Input: part model. Units: mm. Frame: model coordinates. A direction names the side the tool comes from. Round coordinates to 2 decimals unless told otherwise and drop trailing zeros. Loops run counter-clockwise (first coordinate to the right, second up) from the corner with the lowest first, then second, coordinate; pieces in that order, holes last. Notation, with made-up numbers: (83, 26.5) - (91, 26.5) arc R15 cw to (91, 34.5) - close; hole circle Ø9 at (86.25, 26). An arc over 180 degrees is marked (long way). One line per question, with ' | ' between items. Start each with the question number.
from build123d import *

# Parameters (mm, degrees)
F0_W     = 76.2
F0_H     = 76.2
F0_W_2   = 73.025
F0_H_2   = 73.025
F1_DEPTH = 668.3375
F2_R     = 5.08
F3_R     = 5.08
F4_R     = 5.08
F5_R     = 5.08
F6_R     = 5.08
F7_R     = 5.08


with BuildPart() as f1:
    # F0 (on Top) → F1 (new body)
    with BuildSketch(Plane.XY):
        Rectangle(F0_W, F0_H)
        Rectangle(F0_W_2, F0_H_2, mode=Mode.SUBTRACT)
    extrude(amount=F1_DEPTH)

    # F2
    f2_edges = [f1.edges().sort_by_distance(p)[0] for p in [
        (-38.1, -38.1, 334.16875),
    ]]
    fillet(f2_edges, radius=F2_R)

    # F3
    f3_edges = [f1.edges().sort_by_distance(p)[0] for p in [
        (38.1, -38.1, 334.16875),
        (38.1, 38.1, 334.16875),
    ]]
    fillet(f3_edges, radius=F3_R)

    # F4
    f4_edges = [f1.edges().sort_by_distance(p)[0] for p in [
        (-36.5125, 36.5125, 334.16875),
    ]]
    fillet(f4_edges, radius=F4_R)

    # F5
    f5_edges = [f1.edges().sort_by_distance(p)[0] for p in [
        (-38.1, 38.1, 334.16875),
        (36.5125, -36.5125, 334.16875),
    ]]
    fillet(f5_edges, radius=F5_R)

    # F6
    f6_edges = [f1.edges().sort_by_distance(p)[0] for p in [
        (-36.5125, -36.5125, 334.16875),
    ]]
    fillet(f6_edges, radius=F6_R)

    # F7
    f7_edges = [f1.edges().sort_by_distance(p)[0] for p in [
        (36.5125, 36.5125, 334.16875),
    ]]
    fillet(f7_edges, radius=F7_R)


solid = f1.part
(1) Reachability of faces 4 (the face through (38.1, 0, 329)), 5 (the face through (36.512, 0, 329)) from +Z, -Z, +X, -X, +Y, -Y: full face, straight path, thin tool, end or side. Return the list, or none.
(2) Pull-direction query (Y, two-part tool) for faces 1 (the face through (-38.1, 0, 329)), 2 (the face through (-36.512, 0, 329)), 3 (the face through (0, 38.1, 329)); classes: released by +Y, released by -Y, zero draft, split by the parting line, or undercut.
(3) Section A-A, the plane y = 0.5. Output: boundary loops of the cut face in (x, z).
(4) Line query: line 1 along Y through (x, z) = (-24.5, 444); line 2 along X through (y, z) = (35, 199). Output: solid intervals per line, ascending. Write a range as from..to.
(5) Section C-C, the plane z = 69. Output: boundary loops of the cut face in (x, y).
Derived:
1) face 4: +Z, -Z, +X, +Y, -Y | face 5: +Z, -Z
2) face 1: zero draft | face 2: undercut | face 3: released by +Y
3) outline: (-38.1, 0) - (-36.51, 0) - (-36.51, 668.34) - (-38.1, 668.34) - close; (36.51, 0) - (38.1, 0) - (38.1, 668.34) - (36.51, 668.34) - close
4) line 1: y = -38.1..-36.51, 36.51..38.1 | line 2: x = -37.7..-35.05, 35.05..37.7
5) outline: (-38.1, -33.02) arc R5.08 ccw to (-33.02, -38.1) - (33.02, -38.1) arc R5.08 ccw to (38.1, -33.02) - (38.1, 33.02) arc R5.08 ccw to (33.02, 38.1) - (-33.02, 38.1) arc R5.08 ccw to (-38.1, 33.02) - close; hole (-36.51, -31.43) arc R5.08 ccw to (-31.43, -36.51) - (31.43, -36.51) arc R5.08 ccw to (36.51, -31.43) - (36.51, 31.43) arc R5.08 ccw to (31.43, 36.51) - (-31.43, 36.51) arc R5.08 ccw to (-36.51, 31.43) - close
